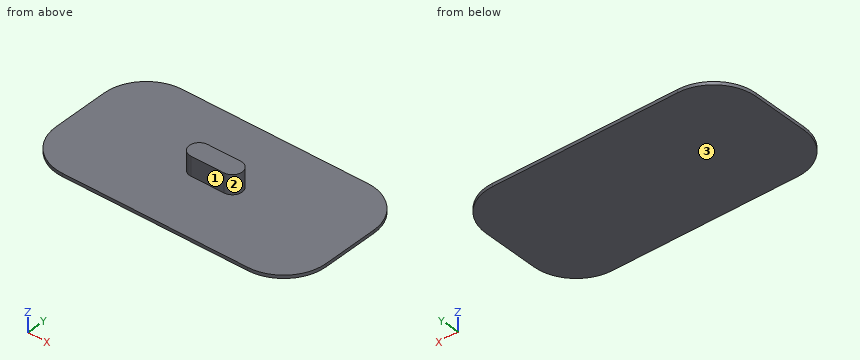
from build123d import *

# Parameters (mm, degrees)
EXTRUDE_1_DEPTH = 3
EXTRUDE_2_DEPTH = 18


with BuildPart() as part:
    # 草图1 → 凸台-拉伸1 (new body)
    with BuildSketch(Plane.XY):
        with BuildLine():
            Line((87.45, 66.5), (-87.45, 66.5))
            ThreePointArc((-87.45, 66.5), (-115.734271247, 54.784271247), (-127.45, 26.5))
            Line((-127.45, 26.5), (-127.45, -26.5))
            ThreePointArc((-127.45, -26.5), (-115.734271247, -54.784271247), (-87.45, -66.5))
            Line((-87.45, -66.5), (87.45, -66.5))
            ThreePointArc((87.45, -66.5), (115.734271247, -54.784271247), (127.45, -26.5))
            Line((127.45, -26.5), (127.45, 26.5))
            ThreePointArc((127.45, 26.5), (115.734271247, 54.784271247), (87.45, 66.5))
        make_face()
    extrude(amount=EXTRUDE_1_DEPTH)

    # 草图2 → 凸台-拉伸2 (add)
    with BuildSketch(Plane.XY.offset(3)):
        with BuildLine():
            Line((-14.821826733, 9.263641708), (16.409879597, 9.263641708))
            ThreePointArc((16.409879597, 9.263641708), (25.673521305, 0), (16.409879597, -9.263641708))
            Line((16.409879597, -9.263641708), (-14.821826733, -9.263641708))
            ThreePointArc((-14.821826733, -9.263641708), (-24.085468441, 0), (-14.821826733, 9.263641708))
        make_face()
    extrude(amount=EXTRUDE_2_DEPTH)


solid = part.part
Could you check a few things on this model? Use its own coordinates, in mm. Face numbers are marked on the shaded views. A direction names the side the tool comes from. Round coordinates to 2 decimals unless told otherwise and drop trailing zeros. Order: outer loops, then holes, each group sorted by start corner. A loop starts at its lowest first (then second) coordinate and runs counter-clockwise, first axis right, second up.
Q1. Imagine slicing it at B-B, the plane x = -58.5. List the corners of the cut face in (y, z) for me.
Geometry says:
outline: (-66.5, 0) - (66.5, 0) - (66.5, 3) - (-66.5, 3) - close
Q2. Please list where these lines run through material, in increasing order: probe 1 along Z at (x, y) = (-0.5, -54.5); probe 2 along Y at (x, z) = (-4, 15); probe 3 along X at (y, z) = (-3, 11.5).
Geometry says:
probe 1: z = 0 to 3
probe 2: y = -9.26 to 9.26
probe 3: x = -23.59 to 25.17
Q3. I'm going to push flat-ended pins straight in: P1, Ø12, axis at y = 13, z = 13.5, coming from the +X side; P2, Ø10, axis at x = 92.5, z = 9.5, coming from the +Y side; P3, Ø6, axis at x = 29.5, y = 52.5, coming from the -Z side; P4, Ø1, axis at x = -75.5, y = -35, coming from the +Z side. Where does each tip first touch, or does it pass through?
Geometry says:
P1: stops at x = 22.48
P2: passes through
P3: stops at z = 0
P4: stops at z = 3
Q4. Imagine slicing it at A-A, the plane y = 0. List the corners of the cut face in (x, z) for me, then the cut area to 3 significant figures.
Geometry says:
outline: (-127.45, 0) - (127.45, 0) - (127.45, 3) - (25.67, 3) - (25.67, 21) - (-24.09, 21) - (-24.09, 3) - (-127.45, 3) - close
area: 1,660 mm2
Q5. Which directions (+Z, -Z, +X, -X, +Y, -Y) give clear straight access to the entire face, cutting with the end or side of a thin tool? Please do the marked faces 1, 2 and 3.
Geometry says:
face 1: +Z, +X, -X, -Y
face 2: +Z, +X
face 3: -Z, +X, -X, +Y, -Y
Q6. Imagine slicing it at C-C, the plane z = 16.75. List the corners of the cut face in (x, y) for me.
Geometry says:
outline: (-14.82, -9.26) - (16.41, -9.26) arc R9.26 ccw to (16.41, 9.26) - (-14.82, 9.26) arc R9.26 ccw to start
